The model under review builds one solid part; all positions refer to its coordinate system, in mm. Face numbers are marked on the shaded views. A direction names the side the tool comes from. Round coordinates to 2 decimals unless told otherwise and drop trailing zeros. Order: outer loops, then holes, each group sorted by start corner. A loop starts at its lowest first (then second) coordinate and runs counter-clockwise, first axis right, second up.
1) Consider section B-B (z = 3). Give the boundary of the cut face in (x, y).
2) To check wall thickness, follow L1, parallel to Z at x = 3.5, y = -13; L2, parallel to Z at x = -7.5, y = 10; L3, parallel to X at y = -11, z = 10. State the ranges of each line that lie inside material, in increasing order.
3) Clearance check with flat-ended pins moving along their axes: P1, Ø9.5, axis at x = 3, y = 1, coming from the +Z side; P2, Ø20.5, axis at x = 0, y = 0, coming from the -Z side; P3, Ø3, axis at y = -13.5, z = 13, coming from the +X side; P4, Ø1.5, axis at y = -2, z = 12.5, coming from the -X side. State where each tip first meets the part, or that it passes through.
4) Consider section A-A (z = 21.5). Give the boundary of the cut face in (x, y).
5) Machinability: for the marked faces 1 and 2, which of the approach directions +Z, -Z, +X, -X, +Y, -Y give a long, thin tool a straight path to every point of the face, cutting with its end or side? Answer none if there is none.
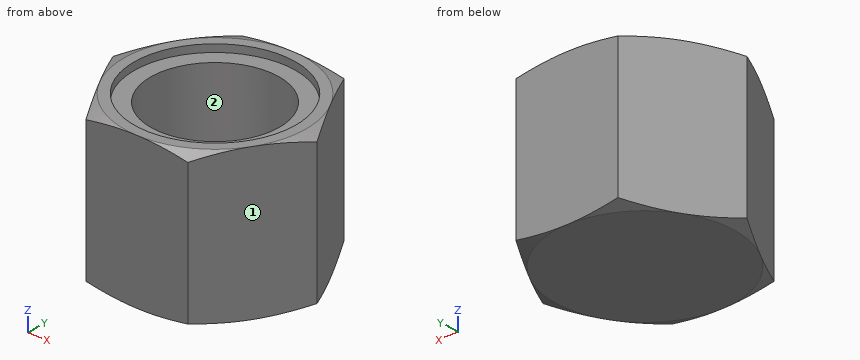
from build123d import *

# Parameters (mm, degrees)
EXTRUDE_1_DEPTH     = 30
SKETCH_2_R          = 12.75
CUT_EXTRUDE_1_DEPTH = 25
SKETCH_3_R          = 13.5
CUT_EXTRUDE_2_DEPTH = 4
SKETCH_4_R          = 16
CUT_EXTRUDE_3_DEPTH = 1.5


with BuildPart() as part:
    # Эскиз1 → Вытянуть1 (new body)
    with BuildSketch(Plane.XY):
        Polygon((10.392304845, 18), (-10.392304845, 18), (-20.784609691, 0), (-10.392304845, -18), (10.392304845, -18), (20.784609691, 0), align=None)
    extrude(amount=EXTRUDE_1_DEPTH)

    # Эскиз2 → Вырез-Вытянуть1 (cut)
    with BuildSketch(Plane.XY.offset(30)):
        Circle(SKETCH_2_R)
    extrude(amount=-CUT_EXTRUDE_1_DEPTH, mode=Mode.SUBTRACT)

    # Эскиз3 → Вырез-Вытянуть2 (cut)
    with BuildSketch(Plane.XY.offset(5)):
        Circle(SKETCH_3_R)
    extrude(amount=CUT_EXTRUDE_2_DEPTH, mode=Mode.SUBTRACT)

    # Эскиз4 → Вырез-Вытянуть3 (cut)
    with BuildSketch(Plane.XY.offset(30)):
        Circle(SKETCH_4_R)
    extrude(amount=-CUT_EXTRUDE_3_DEPTH, mode=Mode.SUBTRACT)

    # Эскиз5 → Вырез-Повернуть1 (revolve, cut)
    with BuildSketch(Plane(origin=(0, 0, 0), x_dir=(1, 0, 0), z_dir=(0, 1, 0))):
        Polygon((20.784609691, -30), (20.784609691, -29), (18, -30), align=None)
        Polygon((20.784609691, 0), (18, 0), (20.784609691, -1), align=None)
    revolve(axis=Axis((0, 0, 28.5), (0, 0, -1)), mode=Mode.SUBTRACT)


solid = part.part
Answer below:
1. outline: (-20.78, 0) - (-10.39, -18) - (10.39, -18) - (20.78, 0) - (10.39, 18) - (-10.39, 18) - close
2. L1: z = 0 to 5, 9 to 28.5
2. L2: z = 0 to 5
2. L3: x = -14.43 to -6.45, 6.45 to 14.43
3. P1: stops at z = 5
3. P2: stops at z = 0
3. P3: stops at x = 13.86
3. P4: stops at x = -20.06
4. outline: (-20.78, 0) - (-10.39, -18) - (10.39, -18) - (20.78, 0) - (10.39, 18) - (-10.39, 18) - close; hole circle Ø25.5 at (0, 0)
5. face 1: +Z, -Z, +X, -Y
5. face 2: +Z
